Geometry check sheet. Reference: the model listing, model coordinates, mm. A direction names the side the tool comes from. Round coordinates to 2 decimals unless told otherwise and drop trailing zeros. Write each loop counter-clockwise with the first axis right and the second up, starting at its lowest first coordinate (ties: lowest second). Pieces come first, ordered by that corner, then holes. Notation, with made-up numbers: M 3.5,3.25 L 45.5,3.25 A32 cw 45.5,41.25 Z; hole C 28.25,32 d7. An arc over 180 degrees is marked long. Put each result on its own line as item: value. Start each with the question number.
(1) Section check B-B on z = 1.6. Record the cut outline in (x, y), then the cut area to 3 significant figures.
(2) Tool access check on faces 1 (the flat face through (-1.5, 0.5, 0.5)), 2 (the cylindrical face through (-1.27, 4.4, 1.77)), 3 (the flat face through (1, 2, -3)), 4 (the flat face through (-2, 4, 0.5)). Record the directions out of +Z, -Z, +X, -X, +Y, -Y that give a thin tool (end or side, any length) a straight path to the whole face; none if there is none.
(3) Gauge pin test, flat ends, axial feed: pin 1 (3 mm diameter, centred on x = -1, z = 2, fed in from -Y); pin 2 (1.5 mm diameter, centred on x = -1, y = 3.5, fed in from -Z); pin 3 (1.5 mm diameter, centred on x = 0, z = -1, fed in from +Y). Record the tip position at first contact, or that the pin passes through.
(4) Section check A-A on y = 3.8. Record the cut outline in (x, z).
(5) Material ranges on probe 1 along Z at (x, y) = (-2.45, 4.1); probe 2 along X at (y, z) = (0.3, 1.5); probe 3 along X at (y, z) = (4, 1.15), recorded low to high.
(6) Section check D-D on y = 2.3. Record the cut outline in (x, z).
(7) Section check C-C on x = 0.4. Record the cut outline in (y, z), then the cut area to 3 significant figures.
from build123d import *

# Parameters (mm, degrees)
SKETCH1_W           = 6
SKETCH1_H           = 6
BOSS_EXTRUDE1_DEPTH = 5
CUT_EXTRUDE7_DEPTH  = 12.5
CUT_EXTRUDE8_DEPTH  = 3.5
SKETCH10_W          = 3
SKETCH10_H          = 1
CUT_EXTRUDE9_DEPTH  = 2.5


with BuildPart() as part:
    # Sketch1 → Boss-Extrude1 (new body)
    with BuildSketch(Plane(origin=(0, 0, 0), x_dir=(1, 0, 0), z_dir=(0, 1, 0))):
        Rectangle(SKETCH1_W, SKETCH1_H)
    extrude(amount=BOSS_EXTRUDE1_DEPTH)

    # Sketch8 → Cut-Extrude7 (cut)
    with BuildSketch(Plane.XY.offset(3)):
        with BuildLine():
            ThreePointArc((0, 3), (1.571067812, 3.893398282), (3, 5))
            Line((3, 5), (-3, 5))
            ThreePointArc((-3, 5), (-1.245414444, 4.381878334), (0, 3))
        make_face()
    extrude(amount=-CUT_EXTRUDE7_DEPTH, mode=Mode.SUBTRACT)

    # Sketch9 → Cut-Extrude8 (cut)
    with BuildSketch(Plane(origin=(0, 0, -3), x_dir=(-1, 0, 0), z_dir=(0, 0, -1))):
        with BuildLine():
            ThreePointArc((0, 3), (1.468871126, 2.406613378), (3, 2))
            Line((3, 2), (3, 5))
            ThreePointArc((3, 5), (1.245414444, 4.381878334), (0, 3))
        make_face()
    extrude(amount=-CUT_EXTRUDE8_DEPTH, mode=Mode.SUBTRACT)

    # Sketch10 → Cut-Extrude9 (cut)
    with BuildSketch(Plane.XY.offset(3)):
        with Locations((-1.5, 0.5)):
            Rectangle(SKETCH10_W, SKETCH10_H)
    extrude(amount=-CUT_EXTRUDE9_DEPTH, mode=Mode.SUBTRACT)


solid = part.part
Answers follow:
1. outline: M -3,1 L 0,1 L 0,0 L 3,0 L 3,5 A12.75 cw 0,3 A3.77 ccw -3,5 Z
1. area: 21.8 mm^2
2. face 1: +Z, -X, -Y
2. face 2: +Z, -Z, +Y
2. face 3: -Z, +X, -X, +Y, -Y
2. face 4: -Z, -X, +Y
3. pin 1: stops at y = 0
3. pin 2: stops at z = 0.5
3. pin 3: stops at y = 3.39
4. outline: M -3,0.5 L -0.56,0.5 L -0.56,3 L -3,3 Z; M 1.43,-3 L 3,-3 L 3,3 L 1.43,3 Z
5. probe 1: z = 0.5 to 3
5. probe 2: x = 0 to 3
5. probe 3: x = -3 to -0.76, 1.73 to 3
6. outline: M -3,0.5 L -1.8,0.5 L -1.8,-3 L 3,-3 L 3,3 L -3,3 Z
7. outline: M 0,-3 L 3.2,-3 L 3.2,3 L 0,3 Z
7. area: 19.2 mm^2
